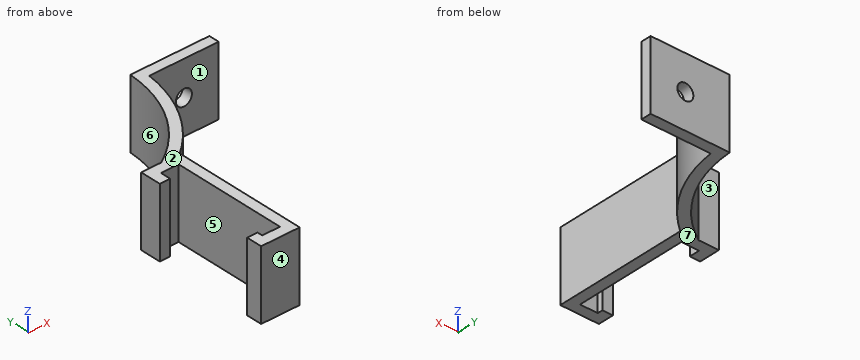
```python
from build123d import *

# Parameters (mm, degrees)
F1_DEPTH = 25.4
F2_R     = 2.921
F3_DEPTH = 87.25


with BuildPart() as f1:
    # F0 (on Top) → F1 (new body)
    with BuildSketch(Plane.XY):
        with BuildLine():
            Line((-24.8285, 20.1295), (-18.3515, 20.1295))
            Line((-18.3515, 20.1295), (-18.3515, -21.3995))
            Line((-18.3515, -21.3995), (-24.8285, -21.3995))
            Line((-24.8285, -21.3995), (-24.8285, -19.4945))
            Line((-24.8285, -19.4945), (-28.6385, -19.4945))
            Line((-28.6385, -19.4945), (-28.6385, -25.2095))
            Line((-28.6385, -25.2095), (-14.5415, -25.2095))
            Line((-14.5415, -25.2095), (-14.5415, 20.1295))
            Line((-14.5415, 20.1295), (-14.5415, 23.9395))
            ThreePointArc((-14.5415, 23.9395), (-1.365036, 39.123287), (4.8895, 58.2295))
            Line((4.8895, 58.2295), (30.2895, 58.2295))
            Line((30.2895, 58.2295), (30.2895, 62.0395))
            Line((30.2895, 62.0395), (1.37959, 62.0395))
            ThreePointArc((1.37959, 62.0395), (-5.1744, 40.149819), (-21.27839, 23.9395))
            Line((-21.27839, 23.9395), (-28.6385, 23.9395))
            Line((-28.6385, 23.9395), (-28.6385, 16.3195))
            Line((-28.6385, 16.3195), (-24.8285, 16.3195))
            Line((-24.8285, 16.3195), (-24.8285, 20.1295))
        make_face()
    extrude(amount=F1_DEPTH)

    # F2 (on face) → F3 (cut, through all)
    with BuildSketch(Plane(origin=(0, 62.0395, 0), x_dir=(-1, 0, 0), z_dir=(0, 1, 0))):
        with Locations((-17.5895, 12.7)):
            Circle(F2_R)
    extrude(amount=-F3_DEPTH, mode=Mode.SUBTRACT)


solid = f1.part
```
Geometry check sheet. Reference: the model listing, model coordinates, mm. Face numbers are marked on the shaded views. A direction names the side the tool comes from. Coordinates: 2 decimals unless noted, no trailing zeros. Write each loop counter-clockwise with the first axis right and the second up, starting at its lowest first coordinate (ties: lowest second). Pieces come first, ordered by that corner, then holes. Notation, with made-up numbers: M -28.5,24.25 L 8.5,24.25 A27 ccw 8.5,46.25 Z; hole C -37,61 d10. An arc over 180 degrees is marked long. One line per item, written item: value. Start each with the question number.
(1) Tool access check on the marked faces 1, 2 and 3. Record the directions out of +Z, -Z, +X, -X, +Y, -Y that give a thin tool (end or side, any length) a straight path to the whole face; none if there is none.
(2) Depth check by flat-ended pin: pin 1 (1.9 mm diameter, centred on x = -27, z = 17.5, fed in from +Y); pin 2 (10 mm diameter, centred on x = 23, z = 15.5, fed in from -Y); pin 3 (0.6 mm diameter, centred on y = -20, z = 11.5, fed in from +X). Enter the tip coordinate at first touch or a pass-through.
(3) Release check for a two-part mould opening along Y. For the marked faces 4, 5, 6 and 7 record: released by +Y, released by -Y, zero draft, split by the parting line, or undercut.
(4) Scan lines: line 1 along X through (y, z) = (10, 23.25); line 2 along Y through (x, z) = (16, 18.5); line 3 along X through (y, z) = (58.5, 11). Record each from-to range of solid material in increasing order. Write a range as [from, to].
(5) Sectioned sample at D-D, the plane y = 14. Enter the section's corners in (x, z), and give its area (3 significant figures).
(6) Sectioned sample at B-B, the plane z = 22.25. Enter the section's corners in (x, y).
(7) Sectioned sample at A-A, the plane z = 12.7. Enter the section's corners in (x, y), and give its area (3 significant figures).
(8) Sectioned sample at C-C, the plane x = -19.5. Enter the section's corners in (y, z).
Filled sheet:
1. face 1: +Z, -Z, +X, -Y
1. face 2: +Z, +X, -X, +Y, -Y
1. face 3: +Z, -Z, -X, +Y
2. pin 1: y = 23.94
2. pin 2: y = 58.23
2. pin 3: x = -14.54
3. face 4: released by -Y
3. face 5: undercut
3. face 6: released by +Y
3. face 7: zero draft
4. line 1: [-18.35, -14.54]
4. line 2: [58.23, 62.04]
4. line 3: [1.08, 15.21], [19.96, 30.29]
5. outline: M -18.35,0 L -14.54,0 L -14.54,25.4 L -18.35,25.4 Z
5. area: 96.8 mm²
6. outline: M -28.64,-25.21 L -14.54,-25.21 L -14.54,23.94 A50.8 ccw 4.89,58.23 L 30.29,58.23 L 30.29,62.04 L 1.38,62.04 A46.99 cw -21.28,23.94 L -28.64,23.94 L -28.64,16.32 L -24.83,16.32 L -24.83,20.13 L -18.35,20.13 L -18.35,-21.4 L -24.83,-21.4 L -24.83,-19.49 L -28.64,-19.49 Z
7. outline: M -28.64,-25.21 L -14.54,-25.21 L -14.54,23.94 A50.8 ccw 4.89,58.23 L 14.67,58.23 L 14.67,62.04 L 1.38,62.04 A46.99 cw -21.28,23.94 L -28.64,23.94 L -28.64,16.32 L -24.83,16.32 L -24.83,20.13 L -18.35,20.13 L -18.35,-21.4 L -24.83,-21.4 L -24.83,-19.49 L -28.64,-19.49 Z; M 20.51,58.23 L 30.29,58.23 L 30.29,62.04 L 20.51,62.04 Z
7. area: 533 mm²
8. outline: M -25.21,0 L -21.4,0 L -21.4,25.4 L -25.21,25.4 Z; M 20.13,0 L 25.07,0 L 25.07,25.4 L 20.13,25.4 Z
